```python
from build123d import *

# Parameters (mm, degrees)
F0_R        = 2.5
F0_W        = 4.0654889308
F0_H        = 4.077391699
F1_DEPTH    = 40
F2_DEPTH    = 0.1
F3_W        = 37.3762528179
F3_H        = 4.5243166387
F4_DEPTH    = 0.8
F5_T1_DEPTH = 61.1957339443
F5_T3_DEPTH = 69.4870657294
F5_T5_DEPTH = 6.3301489651
F5_T7_DEPTH = 53.3325486423
F5_T9_DEPTH = 65


# Not quite as in the source:
# - a fillet or chamfer that OpenCascade refuses, or shapes differently, is made with other operations: its cross-section is extruded or revolved along the edge and cut away or added


with BuildPart() as f1:
    # F0 (on Front) → F1 (new body)
    with BuildSketch(Plane.XZ):
        Polygon((-49.8398691416, 21), (-53.3222284913, 0), (0, 0), (26.6024060547, 0), (66.6777715087, 0), (66.6777715087, 32.0019141734), (0, 32.0019141734), (0, 27.3301489651), (0, 26.5009570867), (4.0654889308, 26.5009570867), (4.0654889308, 22.4235653877), (0, 22.4235653877), (0, 21), align=None)
        with Locations((-39.8388169706, 2.6)):
            Circle(F0_R, mode=Mode.SUBTRACT)
        with Locations((52.0384535193, 2.9)):
            Circle(F0_R, mode=Mode.SUBTRACT)
        with Locations((2.0327444654, 24.4622612372)):
            Rectangle(F0_W, F0_H)
        Polygon((0, 27.3301489651), (0, 32.0019141734), (-3.1343069183, 27.3301489651), align=None)
    extrude(amount=F1_DEPTH)

    # F2 (add): a face of the model
    f2_faces = [f1.faces().sort_by_distance(p)[0] for p in [
        (-24.9199345708, -20, 21),
    ]]
    extrude(f2_faces, amount=-F2_DEPTH)

    # F3 (on Right) → F4 (cut)
    with BuildSketch(Plane.YZ):
        with Locations((-20.0095633627, 24.2089927197)):
            Rectangle(F3_W, F3_H)
    extrude(amount=F4_DEPTH, mode=Mode.SUBTRACT)

    # F5: fillet of radius 5 on 7 edges, made by hand

    # F5_s2 → F5_t1 (cut)
    with BuildSketch(Plane.XZ.offset(-10.5978669722)):
        with BuildLine():
            ThreePointArc((-50.5333622544, 16.81796308), (-48.8341558683, 19.8137786643), (-45.6007223527, 21))
            Line((-45.6007223527, 21), (-49.8398691416, 21))
            Line((-49.8398691416, 21), (-50.5333622544, 16.81796308))
        make_face()
    extrude(amount=F5_T1_DEPTH, mode=Mode.SUBTRACT)

    # F5_s4 → F5_t3 (cut)
    with BuildSketch(Plane.XZ.offset(-14.7435328647)):
        with BuildLine():
            ThreePointArc((-52.3574552471, 5.81796308), (-51.2385940097, 1.7665664844), (-47.4248153454, 0))
            Line((-47.4248153454, 0), (-53.3222284913, 0))
            Line((-53.3222284913, 0), (-52.3574552471, 5.81796308))
        make_face()
    extrude(amount=F5_T3_DEPTH, mode=Mode.SUBTRACT)

    # F5_s6 → F5_t5 (cut)
    with BuildSketch(Plane.XY.offset(21)):
        with BuildLine():
            ThreePointArc((5, 0), (1.4644660941, -1.4644660941), (0, -5))
            Line((0, -5), (0, 0))
            Line((0, 0), (5, 0))
        make_face()
        with BuildLine():
            ThreePointArc((5, -40), (1.4644660941, -38.5355339059), (0, -35))
            Line((0, -35), (0, -40))
            Line((0, -40), (5, -40))
        make_face()
    extrude(amount=F5_T5_DEPTH, mode=Mode.SUBTRACT)

    # F5_s8 → F5_t7 (cut)
    with BuildSketch(Plane.XZ.offset(-6.6662743212)):
        with BuildLine():
            ThreePointArc((2.6665097285, 32.0019141734), (0.3136763633, 31.4137363769), (-1.4856032643, 29.7875842356))
            Line((-1.4856032643, 29.7875842356), (0, 32.0019141734))
            Line((0, 32.0019141734), (2.6665097285, 32.0019141734))
        make_face()
    extrude(amount=F5_T7_DEPTH, mode=Mode.SUBTRACT)

    # F5_s10 → F5_t9 (cut)
    with BuildSketch(Plane.XZ.offset(-12.5)):
        with BuildLine():
            ThreePointArc((61.6777715087, 0), (65.2133054146, 1.4644660941), (66.6777715087, 5))
            Line((66.6777715087, 5), (66.6777715087, 0))
            Line((66.6777715087, 0), (61.6777715087, 0))
        make_face()
        with BuildLine():
            ThreePointArc((66.6777715087, 27.0019141734), (65.2133054146, 30.5374480793), (61.6777715087, 32.0019141734))
            Line((61.6777715087, 32.0019141734), (66.6777715087, 32.0019141734))
            Line((66.6777715087, 32.0019141734), (66.6777715087, 27.0019141734))
        make_face()
    extrude(amount=F5_T9_DEPTH, mode=Mode.SUBTRACT)


solid = f1.part
```
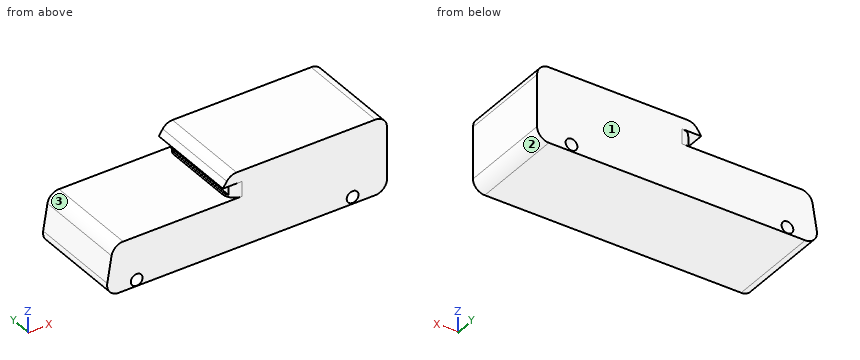
Verification items for the finished model (mm, model axes). Face numbers are marked on the shaded views. Round coordinates to 2 decimals unless told otherwise and drop trailing zeros. Loops run counter-clockwise (first coordinate to the right, second up) from the corner with the lowest first, then second, coordinate; pieces in that order, holes last. Notation, with made-up numbers: (18, 77) -> (42, 77) arc R16 cw to (42, 108) -> close; hole circle Ø4 at (10, 56.25). An arc over 180 degrees is marked (long way). Answer as a JSON object with one key per item and string values.
Q1. Scan lines: line 1 (X direction, y = -32.5, z = 3); line 2 (Z direction, x = 52, y = -27.5); line 3 (Z direction, x = -7.5, y = -37). Record each from-to range of solid material in increasing order. Write a range as from..to.
Data:
{"line 1": "x = -52.01..-42.31, -37.37..49.54, 54.54..66.26", "line 2": "z = 0..0.4, 5.4..32", "line 3": "z = 0..21"}
Q2. Section check A-A (y = -8). Record the boundary of the cut face in (x, z).
Data:
{"outline": "(-52.36, 5.82) arc R5 ccw to (-47.42, 0) -> (61.68, 0) arc R5 ccw to (66.68, 5) -> (66.68, 27) arc R5 ccw to (61.68, 32) -> (2.67, 32) arc R5 ccw to (-1.49, 29.79) -> (-3.13, 27.33) -> (0, 27.33) -> (0, 26.47) -> (0.8, 26.47) -> (0.8, 21.95) -> (0, 21.95) -> (0, 21) -> (-45.6, 21) arc R5 ccw to (-50.53, 16.82) -> close; hole circle Ø5 at (-39.84, 2.6); hole circle Ø5 at (52.04, 2.9)"}
Q3. Go/stop test with flat-tipped pins: P1, Ø0.6, axis at x = 0, y = -15, coming from the +Z side; P2, Ø3.5, axis at y = -22.5, z = 23.5, coming from the -X side; P3, Ø1.5, axis at y = -17, z = 24, coming from the -X side. Record where each tip stops, or that it passes through.
Data:
{"P1": "stops at z = 31.41", "P2": "stops at x = 0", "P3": "stops at x = 0.8"}
Q4. Draft check along Z on the marked faces 1, 2 and 3. Enter one of: pulls with the +Z half, pulls with the -Z half, needs draft (parallel to the pull), parting line crosses it, or undercut.
Data:
{"face 1": "needs draft", "face 2": "pulls with the -Z half", "face 3": "pulls with the +Z half"}
Q5. Section check B-B (x = -9.5). Record the boundary of the cut face in (y, z).
Data:
{"outline": "(-40, 0) -> (0, 0) -> (0, 21) -> (-40, 21) -> close"}
